Input: part model. Units: mm. Frame: model coordinates. Face numbers are marked on the shaded views. A direction names the side the tool comes from. Round coordinates to 2 decimals unless told otherwise and drop trailing zeros. Loops run counter-clockwise (first coordinate to the right, second up) from the corner with the lowest first, then second, coordinate; pieces in that order, holes last. Notation, with made-up numbers: (66, 32) -> (107, 32) arc R22 ccw to (107, 65) -> close; hole circle Ø7 at (14.25, -25.75). An arc over 180 degrees is marked (long way). Answer in a Markdown table with one row per item. Add a question column.
Q1. Section C-C, the plane z = -9. Give the number of separate pieces and of enclosed holes in the cut face, and give its area (3 significant figures).
Q2. Section B-B, the plane x = 25.5. Output: boundary loops of the cut face in (y, z).
Q3. Section D-D, the plane x = 49.5. Output: boundary loops of the cut face in (y, z).
Q4. Mould query, pull axis X, two halves, no side actions, for the marked faces 5 and 6. Classes: pulls with the +X half, pulls with the -X half, needs draft (parallel to the pull), parting line crosses it, or undercut.
Q5. Reachability of the marked faces 1, 2, 3 and 4 from +Z, -Z, +X, -X, +Y, -Y: full face, straight path, thin tool, end or side. Return the list, or none.
Q6. Section A-A, the plane y = 22.5. Output: boundary loops of the cut face in (x, z).
Q7. Pin query (flat end, axial travel): pin 1 (5.5 mm diameter, centred on x = 67, y = 18, fed in from +Z); pin 2 (2.5 mm diameter, centred on y = 36, z = -10, fed in from +X); pin 3 (2 mm diameter, centred on x = 65.5, y = 16, fed in from -Z). Return the tip coordinate at first contact, or that it passes through.
Q8. Ray query, L1, parallel to Z at x = 59.12, y = 1.55; L2, parallel to Y at x = 10.5, z = -6; L3, parallel to X at y = 36, z = -19. Return the intervals inside material, ascending. Write a range as from..to.
```python
from build123d import *

# Parameters (mm, degrees)
ESQUISSE1_W                                    = 90
ESQUISSE1_H                                    = 33
BOSS_EXTRU_1_DEPTH                             = 4
ESQUISSE2_R                                    = 1.5
ENL_V_MAT_EXTRU_1_DEPTH                        = 4
ESQUISSE3_W                                    = 10
ESQUISSE3_H                                    = 10
BOSS_EXTRU_2_DEPTH                             = 31
ESQUISSE4_W                                    = 20
ESQUISSE4_H                                    = 33
BOSS_EXTRU_3_DEPTH                             = 3
CONG_1_R                                       = 4
FRAISAGE_POUR_VIS_T_TE_FRAIS_E_M31_D           = 3.4
FRAISAGE_POUR_VIS_T_TE_FRAIS_E_M31_DEPTH       = 10
FRAISAGE_POUR_VIS_T_TE_FRAIS_E_M31_CSINK_D     = 6.3
FRAISAGE_POUR_VIS_T_TE_FRAIS_E_M31_CSINK_ANGLE = 90
FRAISAGE_POUR_VIS_T_TE_FRAIS_E_M31_TIP         = 1.021463052
CONG_2_R                                       = 3


with BuildPart() as part:
    # Esquisse1 → Boss.-Extru.1 (new body)
    with BuildSketch(Plane(origin=(0, 0, 0), x_dir=(1, 0, 0), z_dir=(0, 1, 0))):
        with Locations((45, 16.5)):
            Rectangle(ESQUISSE1_W, ESQUISSE1_H)
    extrude(amount=BOSS_EXTRU_1_DEPTH)

    # Esquisse2 → Enlèv. mat.-Extru.1 (cut)
    with BuildSketch(Plane(origin=(0, 4, 0), x_dir=(1, 0, 0), z_dir=(0, 1, 0))):
        with Locations(Location((20, 29.2, 0), (0, 0, 270))):
            Circle(ESQUISSE2_R)
        with Locations(Location((59.12, 29.2, 0), (0, 0, 270))):
            Circle(ESQUISSE2_R)
        with Locations(Location((59.12, 3.8, 0), (0, 0, 270))):
            Circle(ESQUISSE2_R)
        with Locations(Location((20, 3.8, 0), (0, 0, 270))):
            Circle(ESQUISSE2_R)
    extrude(amount=-ENL_V_MAT_EXTRU_1_DEPTH, mode=Mode.SUBTRACT)

    # Esquisse3 → Boss.-Extru.2 (add)
    with BuildSketch(Plane(origin=(0, 4, 0), x_dir=(1, 0, 0), z_dir=(0, 1, 0))):
        with Locations((22, 16.5)):
            Rectangle(ESQUISSE3_W, ESQUISSE3_H)
        with Locations((68, 16.5)):
            Rectangle(ESQUISSE3_W, ESQUISSE3_H)
    extrude(amount=BOSS_EXTRU_2_DEPTH)

    # Esquisse4 → Boss.-Extru.3 (add)
    with BuildSketch(Plane(origin=(0, 35, 0), x_dir=(1, 0, 0), z_dir=(0, 1, 0))):
        with Locations((17, 16.5)):
            Rectangle(ESQUISSE4_W, ESQUISSE4_H)
        with Locations((73, 16.5)):
            Rectangle(ESQUISSE4_W, ESQUISSE4_H)
    extrude(amount=BOSS_EXTRU_3_DEPTH)

    # Congé1
    cong_1_edges = [part.edges().sort_by_distance(p)[0] for p in [
        (22, 4, -11.5),
        (27, 4, -16.5),
        (22, 4, -21.5),
        (63, 4, -16.5),
        (68, 4, -11.5),
        (68, 4, -21.5),
        (0, 2, -33),
        (90, 2, -33),
        (90, 2, 0),
        (0, 2, 0),
    ]]
    fillet(cong_1_edges, radius=CONG_1_R)

    # Fraisage pour vis à tête fraisée M31
    with Locations(Plane(origin=(0, 4, 0), x_dir=(1, 0, 0), z_dir=(0, 1, 0))):
        with Locations((59.12, 3.8), (59.12, 29.2), (20, 3.8), (20, 29.2)):
            CounterSinkHole(FRAISAGE_POUR_VIS_T_TE_FRAIS_E_M31_D / 2, FRAISAGE_POUR_VIS_T_TE_FRAIS_E_M31_CSINK_D / 2, depth=FRAISAGE_POUR_VIS_T_TE_FRAIS_E_M31_DEPTH, counter_sink_angle=FRAISAGE_POUR_VIS_T_TE_FRAIS_E_M31_CSINK_ANGLE)
            with Locations((0, 0, -(FRAISAGE_POUR_VIS_T_TE_FRAIS_E_M31_DEPTH + FRAISAGE_POUR_VIS_T_TE_FRAIS_E_M31_TIP / 2))):  # 118° drill point
                Cone(0, FRAISAGE_POUR_VIS_T_TE_FRAIS_E_M31_D / 2, FRAISAGE_POUR_VIS_T_TE_FRAIS_E_M31_TIP, mode=Mode.SUBTRACT)

    # Congé2
    # the kernel refuses this fillet: 3 mm, written as the material it takes off along each edge
    with BuildSketch(Plane(origin=(17, 8, -25.5), x_dir=(0, 0, 1), z_dir=(0, 1, 0))) as cong_2_piece_1_section:
        with BuildLine():
            CenterArc((4 + CONG_2_R, CONG_2_R), CONG_2_R, 180, 90)
            Line((4, CONG_2_R), (4, 0))
            Line((4, 0), (4 + CONG_2_R, 0))
        make_face()
    cong_2_piece_1 = revolve(axis=Axis((17, 8, -25.5), (1, 0, 0)), revolution_arc=197.472741928, mode=Mode.PRIVATE)
    cong_2_piece_1 = split(cong_2_piece_1, bisect_by=Plane(origin=(17, 4, -25.5), z_dir=(0, 1, 0)), keep=Keep.TOP, mode=Mode.PRIVATE)
    add(cong_2_piece_1, mode=Mode.SUBTRACT)
    with BuildSketch(Plane(origin=(73, 8, -25.5), x_dir=(0, 0.3002520412299313, -0.9538599015249879), z_dir=(0, 0.9538599015249879, 0.3002520412299313))) as cong_2_piece_2_section:
        with BuildLine():
            CenterArc((4 + CONG_2_R, CONG_2_R), CONG_2_R, 180, 90)
            Line((4, CONG_2_R), (4, 0))
            Line((4, 0), (4 + CONG_2_R, 0))
        make_face()
    cong_2_piece_2 = revolve(axis=Axis((73, 8, -25.5), (-1, 0, 0)), revolution_arc=197.472741928, mode=Mode.PRIVATE)
    cong_2_piece_2 = split(cong_2_piece_2, bisect_by=Plane(origin=(73, 4, -25.5), z_dir=(0, 1, 0)), keep=Keep.TOP, mode=Mode.PRIVATE)
    add(cong_2_piece_2, mode=Mode.SUBTRACT)
    with BuildSketch(Plane(origin=(73, 8, -7.5), x_dir=(0, 0.30025204122993077, 0.9538599015249881), z_dir=(0, 0.9538599015249881, -0.30025204122993077))) as cong_2_piece_3_section:
        with BuildLine():
            CenterArc((4 + CONG_2_R, -CONG_2_R), CONG_2_R, 90, 90)
            Line((4, -CONG_2_R), (4, 0))
            Line((4, 0), (4 + CONG_2_R, 0))
        make_face()
    cong_2_piece_3 = revolve(axis=Axis((73, 8, -7.5), (1, 0, 0)), revolution_arc=197.472741928, mode=Mode.PRIVATE)
    cong_2_piece_3 = split(cong_2_piece_3, bisect_by=Plane(origin=(73, 4, -7.5), z_dir=(0, 1, 0)), keep=Keep.TOP, mode=Mode.PRIVATE)
    add(cong_2_piece_3, mode=Mode.SUBTRACT)
    with BuildSketch(Plane(origin=(17, 8, -7.5), x_dir=(0, 0, -1), z_dir=(0, 1, 0))) as cong_2_piece_4_section:
        with BuildLine():
            CenterArc((4 + CONG_2_R, -CONG_2_R), CONG_2_R, 90, 90)
            Line((4, -CONG_2_R), (4, 0))
            Line((4, 0), (4 + CONG_2_R, 0))
        make_face()
    cong_2_piece_4 = revolve(axis=Axis((17, 8, -7.5), (-1, 0, 0)), revolution_arc=197.472741928, mode=Mode.PRIVATE)
    cong_2_piece_4 = split(cong_2_piece_4, bisect_by=Plane(origin=(17, 4, -7.5), z_dir=(0, 1, 0)), keep=Keep.TOP, mode=Mode.PRIVATE)
    add(cong_2_piece_4, mode=Mode.SUBTRACT)
    with BuildSketch(Plane(origin=(17, 8, -21.5), x_dir=(0, 0, 1), z_dir=(0, 1, 0)), Plane(origin=(17, 8, -11.5), x_dir=(1, 0, 0), z_dir=(0, 1, 0)), Plane(origin=(73, 8, -11.5), x_dir=(0, 0, -1), z_dir=(0, 1, 0))) as cong_2_piece_5:
        with BuildLine():
            CenterArc((CONG_2_R, CONG_2_R), CONG_2_R, 180, 90)
            Line((0, CONG_2_R), (0, 0))
            Line((0, 0), (CONG_2_R, 0))
        make_face()
    extrude(amount=27, mode=Mode.SUBTRACT)
    with BuildSketch(Plane(origin=(73, 8, -21.5), x_dir=(0, 0, 1), z_dir=(0, 1, 0))) as cong_2_piece_6:
        with BuildLine():
            CenterArc((CONG_2_R, -CONG_2_R), CONG_2_R, 90, 90)
            Line((0, -CONG_2_R), (0, 0))
            Line((0, 0), (CONG_2_R, 0))
        make_face()
    extrude(amount=27, mode=Mode.SUBTRACT)


solid = part.part
```
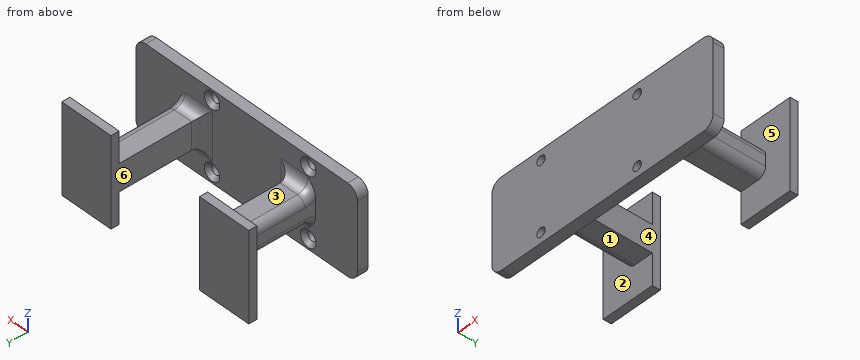
Answer block:
| question | item | result |
|---|---|---|
| 1 | separate pieces | 3 |
| 1 | enclosed holes | 0 |
| 1 | area | 486 mm^2 |
| 2 | outline | (0, -33) -> (4, -33) -> (4, -25.5) arc R4 cw to (8, -21.5) -> (35, -21.5) -> (35, -33) -> (38, -33) -> (38, 0) -> (35, 0) -> (35, -11.5) -> (8, -11.5) arc R4 cw to (4, -7.5) -> (4, 0) -> (0, 0) -> close |
| 3 | outline | (0, -33) -> (4, -33) -> (4, 0) -> (0, 0) -> close |
| 4 | face 5 | needs draft |
| 4 | face 6 | undercut |
| 5 | face 1 | -Z, +X, -X |
| 5 | face 2 | -X |
| 5 | face 3 | +Z, +X, -X |
| 5 | face 4 | +Z, -Z, +Y |
| 6 | outline | (17, -18.5) arc R3 ccw to (20, -21.5) -> (27, -21.5) -> (27, -11.5) -> (20, -11.5) arc R3 ccw to (17, -14.5) -> close; (63, -21.5) -> (70, -21.5) arc R3 ccw to (73, -18.5) -> (73, -14.5) arc R3 ccw to (70, -11.5) -> (63, -11.5) -> close |
| 7 | pin 1 | z = -11.5 |
| 7 | pin 2 | x = 83 |
| 7 | pin 3 | z = -21.5 |
| 8 | L1 | -33..-30.9, -27.5..-5.5, -2.1..0 |
| 8 | L2 | 0..4, 35..38 |
| 8 | L3 | 7..27, 63..83 |
